Geometry check sheet. Reference: drawing and pictorial views, mm from the part's lowest x, y, z. A direction names the side the tool comes from. Round coordinates to 2 decimals unless told otherwise and drop trailing zeros. Order: outer loops, then holes, each group sorted by start corner. A loop starts at its lowest first (then second) coordinate and runs counter-clockwise, first axis right, second up.
(1) Set-up check for the marked faces 1 and 2: record each of +Z, -Z, +X, -X, +Y, -Y from which the full face is reachable in a straight line by a thin tool's end or side.
(2) Release check for a two-part mould opening along Z. For the marked faces 3, 4, 5 and 6 record: +Z half, -Z half, draft (parallel to the pull), parting line (faces both ways), or undercut.
(3) Sectioned sample at D-D (y = 7). Record the boundary of the cut face in (x, z), plus the area to 3 significant figures.
(4) Sectioned sample at A-A (z = 9). Record the boundary of the cut face in (x, y).
(5) Sectioned sample at B-B (y = 1.75). Give the number of separate pieces and of enclosed holes in the cut face, plus the area to 3 significant figures.
(6) Material ranges on line 1 along Z through (x, y) = (4, 2.1) (1 decimal); line 2 along X through (y, z) = (3, 24); line 3 along X through (y, z) = (2.5, 4) (1 decimal), recorded low to high.
(7) Sectioned sample at C-C (x = 4). Record the boundary of the cut face in (y, z) (1 decimal).
(8) Go/stop test with a flat-tipped pin: pin 1 (4 mm diameter, centred on x = 4, z = 4, fed in from +Y). Record where the tip stops, or that it passes through.
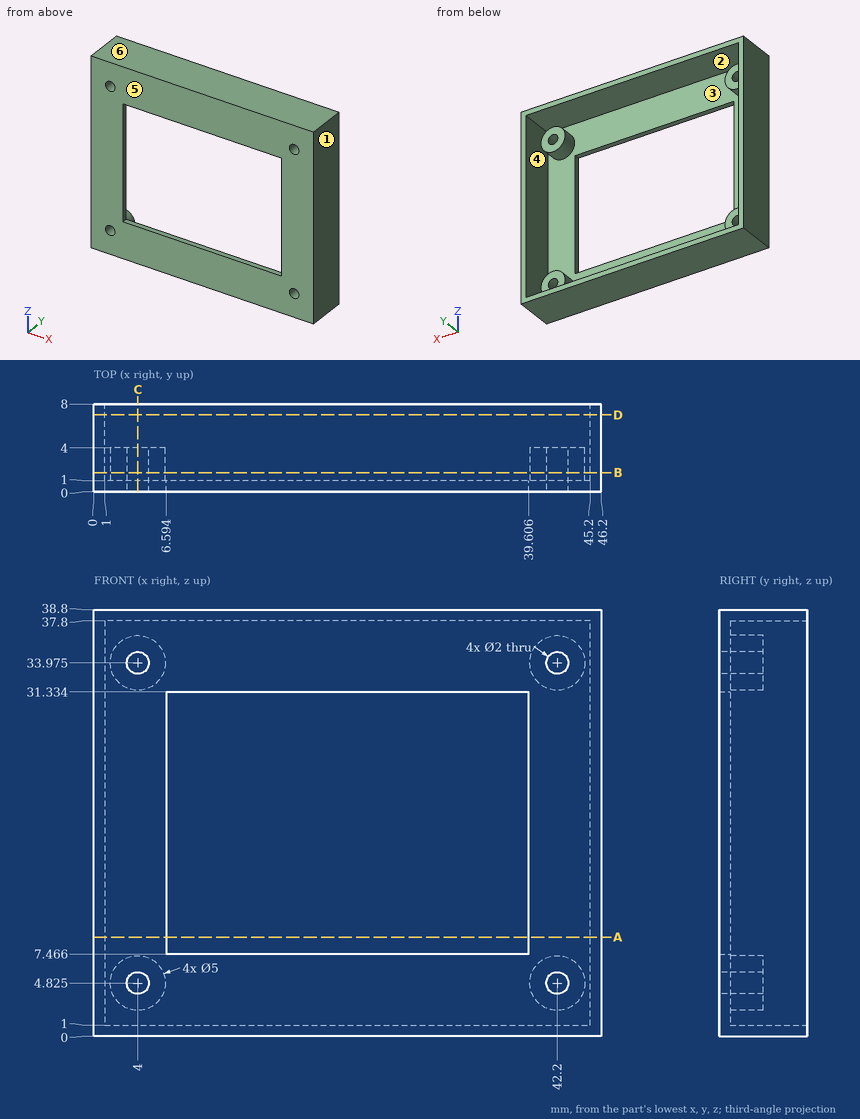
Answer below:
1. face 1: +Z, -Z, +X, +Y, -Y
1. face 2: +Y
2. face 3: undercut
2. face 4: undercut
2. face 5: draft
2. face 6: +Z half
3. outline: (0, 0) - (46.2, 0) - (46.2, 38.8) - (0, 38.8) - close; hole (1, 1) - (45.2, 1) - (45.2, 37.8) - (1, 37.8) - close
3. area: 166 mm2
4. outline: (0, 0) - (6.59, 0) - (6.59, 1) - (1, 1) - (1, 8) - (0, 8) - close; (39.61, 0) - (46.2, 0) - (46.2, 8) - (45.2, 8) - (45.2, 1) - (39.61, 1) - close
5. separate pieces: 5
5. enclosed holes: 5
5. area: 232 mm2
6. line 1: z = 0 to 1, 2.3 to 3.8, 5.8 to 7.3, 31.5 to 33, 35 to 36.5, 37.8 to 38.8
6. line 2: x = 0 to 1, 45.2 to 46.2
6. line 3: x = 0 to 1, 1.6 to 3.4, 4.6 to 6.4, 39.8 to 41.6, 42.8 to 44.6, 45.2 to 46.2
7. outline: (0, 0) - (8, 0) - (8, 1) - (1, 1) - (1, 2.3) - (4, 2.3) - (4, 3.8) - (0, 3.8) - close; (0, 5.8) - (4, 5.8) - (4, 7.3) - (1, 7.3) - (1, 31.5) - (4, 31.5) - (4, 33) - (0, 33) - close; (0, 35) - (4, 35) - (4, 36.5) - (1, 36.5) - (1, 37.8) - (8, 37.8) - (8, 38.8) - (0, 38.8) - close
8. pin 1: stops at y = 4
